from build123d import *

# Parameters (mm, degrees)
SKETCH2_W                  = 125
SKETCH2_H                  = 96
SKETCH2_R                  = 8
SKETCH2_R_2                = 19.1
BOSS_EXTRUDE1_DEPTH        = 30
M4X0_7_TAPPED_HOLE1_D      = 3.3
SKETCH10_W                 = 96
SKETCH10_H                 = 30
BOSS_EXTRUDE3_DEPTH        = 2
M6X1_0_TAPPED_HOLE1_D      = 5
M6X1_0_TAPPED_HOLE1_DEPTH  = 11
M6X1_0_TAPPED_HOLE1_TIP    = 1.502151548
M6X1_0_TAPPED_HOLE3_REACH  = 121.483
M6X1_0_TAPPED_HOLE3_BORE_R = 2.5
FILLET1_R                  = 2


with BuildPart() as part:
    # Sketch2 → Boss-Extrude1 (new body)
    with BuildSketch(Plane(origin=(0, 0, 0), x_dir=(1, 0, 0), z_dir=(0, 1, 0))):
        Rectangle(SKETCH2_W, SKETCH2_H)
        with Locations(Location((-44, 29, 0), (0, 0, 270))):
            Circle(SKETCH2_R, mode=Mode.SUBTRACT)
        with Locations(Location((-44, -29, 0), (0, 0, 270))):
            Circle(SKETCH2_R, mode=Mode.SUBTRACT)
        with Locations(Location((44, -29, 0), (0, 0, 270))):
            Circle(SKETCH2_R, mode=Mode.SUBTRACT)
        with Locations(Location((44, 29, 0), (0, 0, 270))):
            Circle(SKETCH2_R, mode=Mode.SUBTRACT)
        with Locations(Location((0, 0, 0), (0, 0, 270))):
            Circle(SKETCH2_R_2, mode=Mode.SUBTRACT)
    extrude(amount=BOSS_EXTRUDE1_DEPTH)

    # M4x0.7 Tapped Hole1 (through all)
    with Locations(Plane(origin=(0, 30, 0), x_dir=(1, 0, 0), z_dir=(0, 1, 0))):
        with Locations((-23.5712, 23.5712), (23.5712, 23.5712), (23.5712, -23.5712), (-23.5712, -23.5712)):
            Hole(M4X0_7_TAPPED_HOLE1_D / 2)

    # Sketch10 → Boss-Extrude3 (add)
    with BuildSketch(Plane(origin=(62.5, 0, 0), x_dir=(0, 0, -1), z_dir=(1, 0, 0))):
        with Locations((0, 15)):
            Rectangle(SKETCH10_W, SKETCH10_H)
    extrude(amount=BOSS_EXTRUDE3_DEPTH)

    # M6x1.0 Tapped Hole1
    with Locations(Plane(origin=(64.5, 0, 0), x_dir=(0, 0, -1), z_dir=(1, 0, 0))):
        with Locations((-33, 15), (0, 15), (33, 15)):
            Hole(M6X1_0_TAPPED_HOLE1_D / 2, depth=M6X1_0_TAPPED_HOLE1_DEPTH)
            with Locations((0, 0, -(M6X1_0_TAPPED_HOLE1_DEPTH + M6X1_0_TAPPED_HOLE1_TIP / 2))):  # 118° drill point
                Cone(0, M6X1_0_TAPPED_HOLE1_D / 2, M6X1_0_TAPPED_HOLE1_TIP, mode=Mode.SUBTRACT)

    # M6x1.0 Tapped Hole3 bore → M6x1.0 Tapped Hole3 (cut, up to next)
    with BuildSketch(Plane(origin=(0, 0, -48), x_dir=(-1, 0, 0), z_dir=(0, 0, -1)), mode=Mode.PRIVATE) as m6x1_0_tapped_hole3_sk1:
        with Locations((-44, 15)):
            Circle(M6X1_0_TAPPED_HOLE3_BORE_R)
    m6x1_0_tapped_hole3_tool1 = extrude(m6x1_0_tapped_hole3_sk1.sketch, amount=-M6X1_0_TAPPED_HOLE3_REACH, mode=Mode.PRIVATE) & part.part
    # M6x1.0 Tapped Hole3 bore → M6x1.0 Tapped Hole3 (cut, up to next)
    with BuildSketch(Plane(origin=(0, 0, -48), x_dir=(-1, 0, 0), z_dir=(0, 0, -1)), mode=Mode.PRIVATE) as m6x1_0_tapped_hole3_sk2:
        with Locations((44, 15)):
            Circle(M6X1_0_TAPPED_HOLE3_BORE_R)
    m6x1_0_tapped_hole3_tool2 = extrude(m6x1_0_tapped_hole3_sk2.sketch, amount=-M6X1_0_TAPPED_HOLE3_REACH, mode=Mode.PRIVATE) & part.part
    m6x1_0_tapped_hole3_1 = m6x1_0_tapped_hole3_tool1.solids().sort_by_distance((44, 15, -48))[0]
    add(m6x1_0_tapped_hole3_1, mode=Mode.SUBTRACT)
    m6x1_0_tapped_hole3_2 = m6x1_0_tapped_hole3_tool2.solids().sort_by_distance((-44, 15, -48))[0]
    add(m6x1_0_tapped_hole3_2, mode=Mode.SUBTRACT)
    m6x1_0_tapped_hole3 = m6x1_0_tapped_hole3_1 + m6x1_0_tapped_hole3_2  # M6x1.0 Tapped Hole3 as one shape, for the pattern or mirror that repeats it

    # Fillet1
    fillet1_edges = [part.edges().sort_by_distance(p)[0] for p in [
        (64.5, 15, 48),
        (64.5, 15, -48),
        (-62.5, 15, -48),
        (-62.5, 15, 48),
    ]]
    fillet(fillet1_edges, radius=FILLET1_R)

    # Mirror1: M6x1.0 Tapped Hole3 across plane
    add(m6x1_0_tapped_hole3.mirror(Plane.XY), mode=Mode.SUBTRACT)


solid = part.part
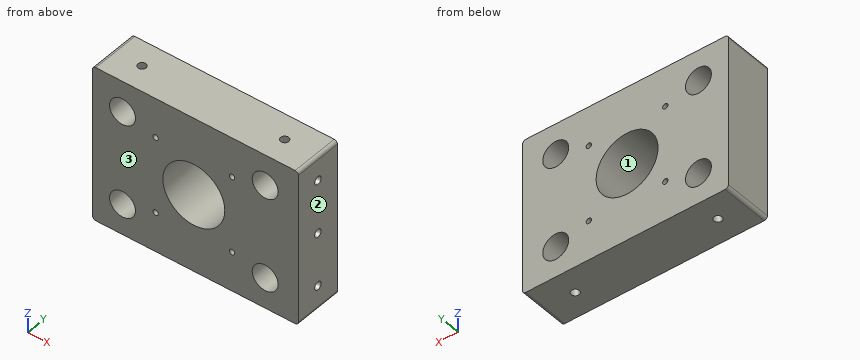
The model under review builds one solid part; all positions refer to its coordinate system, in mm. Face numbers are marked on the shaded views. Coordinates: 2 decimals unless noted, no trailing zeros. Write each loop counter-clockwise with the first axis right and the second up, starting at its lowest first coordinate (ties: lowest second). Pieces come first, ordered by that corner, then holes. Notation, with made-up numbers: M -22.75,3 L 28.25,3 A17 cw 28.25,14 Z; hole C -25,9 d11. An arc over 180 degrees is marked long. Put each result on its own line as item: value.
1) Add section D-D on z = -4.5. Give the boundary of the cut face in (x, y).
Computed:
outline: M -62.5,0 L -18.56,0 L -18.56,30 L -62.5,30 Z; M 18.56,0 L 64.5,0 L 64.5,30 L 18.56,30 Z
2) Wall thickness on probe 1 along Z at (x, y) = (43.5, 10.5); probe 2 along X at (y, z) = (15, 42); probe 3 along X at (y, z) = (18.5, -29): over which ranges is each line inside the solid? List them lowest first. Write a range as [from, to].
Computed:
probe 1: z = [-48, -36.98], [-21.02, 21.02], [36.98, 48]
probe 2: x = [-62.5, -46.5], [-41.5, 41.5], [46.5, 64.5]
probe 3: x = [-62.5, -52], [-36, 36], [52, 64.5]
3) Draft analysis for pull direction X (two halves, no side actions). For the marked faces 1, 2 and 3, state which applies: released by +X, released by -X, zero draft, split by the parting line, or undercut.
Computed:
face 1: undercut
face 2: released by +X
face 3: zero draft
4) Add section B-B on z = 29. Give the boundary of the cut face in (x, y), then the cut area to 3 significant figures.
Computed:
outline: M -62.5,0 L -52,0 L -52,30 L -62.5,30 Z; M -36,0 L 36,0 L 36,30 L -36,30 Z; M 52,0 L 64.5,0 L 64.5,30 L 52,30 Z
area: 2,850 mm2
5) Clearance check with a flat-ended pin moving along its axis: pin 1 Ø4 at (x, y) = (44, 15) entering from +Z. State where the tip first meets the part, or that it passes through.
Computed:
pin 1: stops at z = 21.25
6) Add section C-C on x = -44. Give the boundary of the cut face in (y, z).
Computed:
outline: M 0,-48 L 12.5,-48 L 12.5,-37 L 0,-37 Z; M 0,-21 L 30,-21 L 30,21 L 0,21 Z; M 0,37 L 12.5,37 L 12.5,48 L 0,48 Z; M 17.5,-48 L 30,-48 L 30,-37 L 17.5,-37 Z; M 17.5,37 L 30,37 L 30,48 L 17.5,48 Z
7) Add section A-A on x = 0. Give the boundary of the cut face in (y, z), then the cut area to 3 significant figures.
Computed:
outline: M 0,-48 L 30,-48 L 30,-19.1 L 0,-19.1 Z; M 0,19.1 L 30,19.1 L 30,48 L 0,48 Z
area: 1,730 mm2
